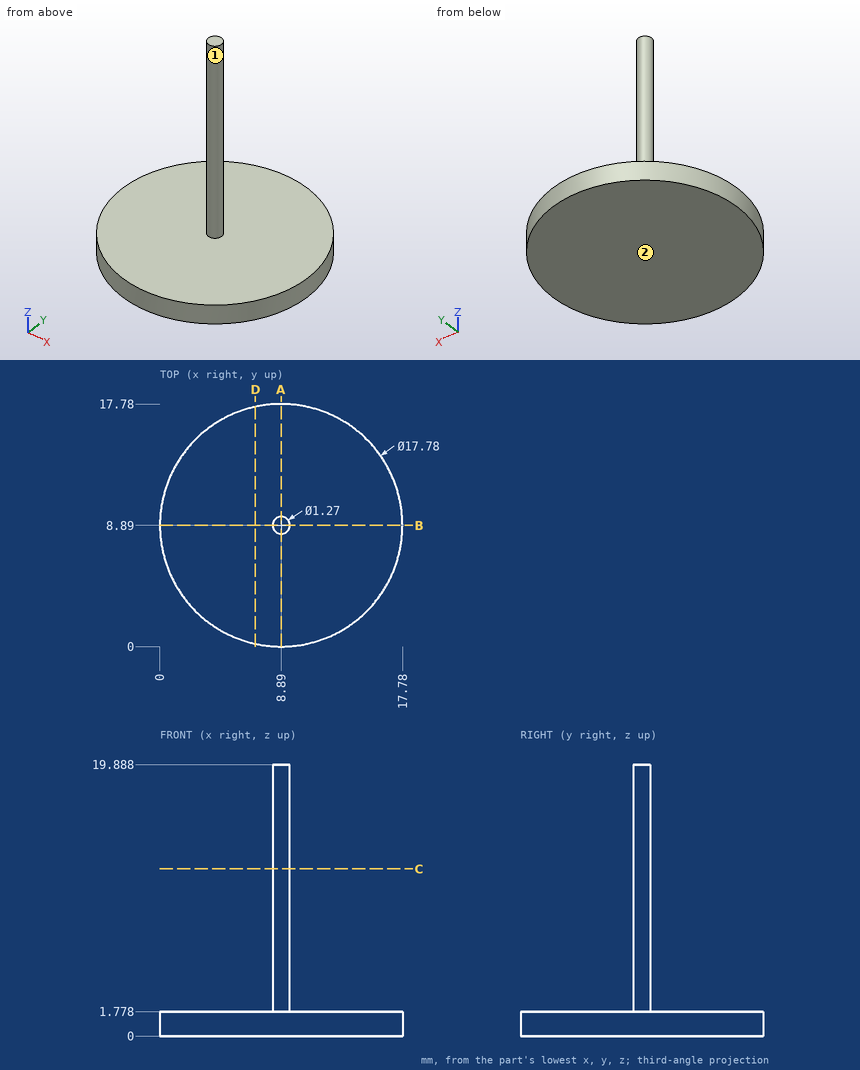
Here's the drawing with two shaded views (mm, measured from the low corner). I have some questions. Give positions to 0.01 mm unless a question says otherwise; leave off trailing zeros. Write each loop counter-clockwise with the first axis right and the second up, starting at its lowest first coordinate (ties: lowest second). Pieces come first, ordered by that corner, then holes. Notation, with made-up numbers: (-30, -12) - (-25, -12) arc R27 ccw to (-25, 23) - close; hole circle Ø5 at (-18.5, 48.25). An arc over 180 degrees is marked (long way). Write item = value, one per line. Start each with the question number.
1. Imagine slicing it at A-A (x = 8.89). Please give me the cut outline in (y, z) (1 decimal).
2. For pin 1 (1 mm diameter, centred on x = 10.5, y = 11.5, fed in from +Z); pin 2 (1.5 mm diameter, centred on x = 6.5, z = 13, fed in from +Y); pin 3 (10 mm diameter, centred on x = 10, z = 16.5, fed in from -Y) (3 decimals); pin 4 (10 mm diameter, centred on x = 6, z = 15, fed in from +Y) (3 decimals), each with a flat end and sliding along its axis, tell me the tip position at first contact or that it passes through.
3. Please list where these lines run through material, in increasing order: line 1 (Z direction, x = 3.25, y = 3); line 2 (X direction, y = 11.5, z = 1.5); line 3 (X direction, y = 4, z = 1.5) (1 decimal).
4. Thinking about a two-plate mould opening in Y: for the marked faces 1 and 2, which applies, released by +Y, released by -Y, zero draft, split by the parting line, or undercut?
5. Imagine slicing it at C-C (z = 12.25). Please give me the cut outline in (x, y) (3 decimals), and give its area (3 significant figures).
6. Imagine slicing it at D-D (x = 7). Please give me the cut outline in (y, z).
Worked answers:
q1.outline = (0, 0) - (17.8, 0) - (17.8, 1.8) - (9.5, 1.8) - (9.5, 19.9) - (8.3, 19.9) - (8.3, 1.8) - (0, 1.8) - close
q2.pin_1 = 1.78
q2.pin_2 = through
q2.pin_3 = 8.255
q2.pin_4 = 9.525
q3.line_1 = 0 to 1.78
q3.line_2 = 0.39 to 17.39
q3.line_3 = 1.5 to 16.3
q4.face_1 = split by the parting line
q4.face_2 = zero draft
q5.outline = circle Ø1.27 at (8.89, 8.89)
q5.area = 1.27 mm2
q6.outline = (0.2, 0) - (17.58, 0) - (17.58, 1.78) - (0.2, 1.78) - close
